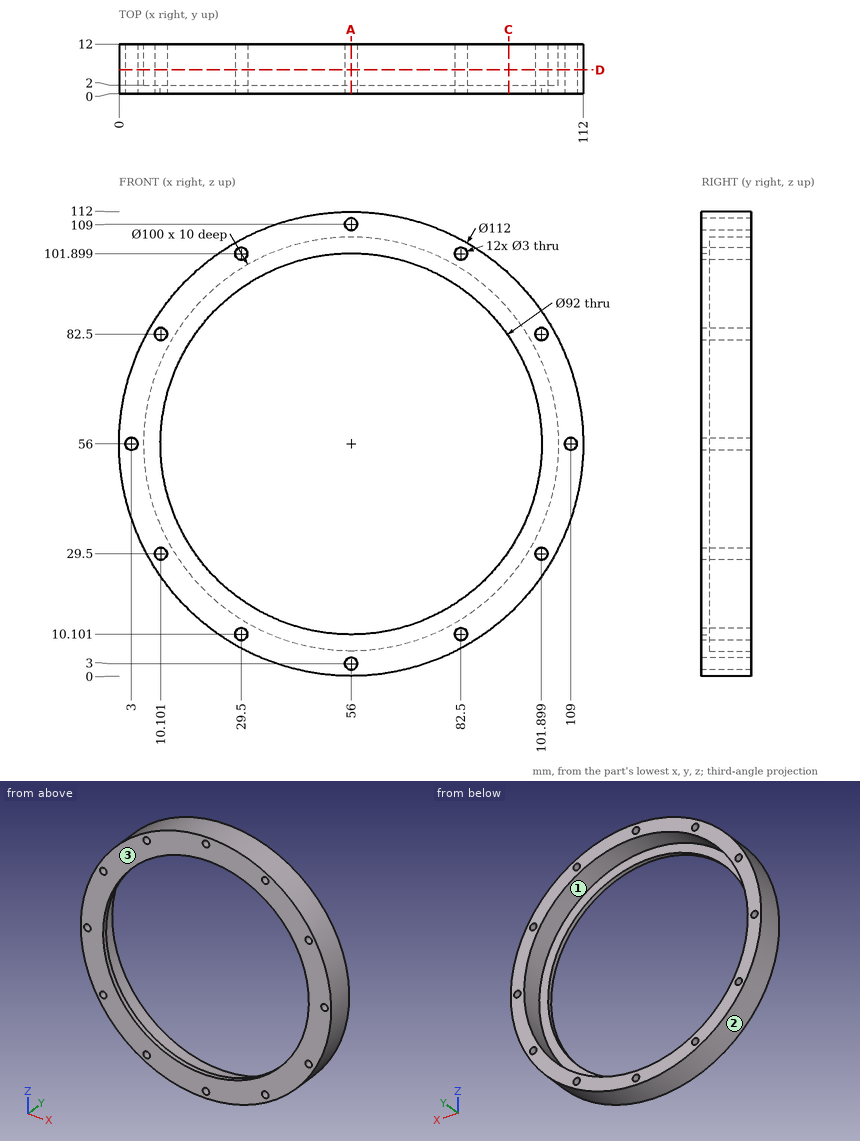
Job drawing, mm, ordinate dimensions from the low corner. One solid piece. Coordinates: 2 decimals unless noted, no trailing zeros. Write each loop counter-clockwise with the first axis right and the second up, starting at its lowest first coordinate (ties: lowest second). Pieces come first, ordered by that corner, then holes.
Item 1: Mould opens along X. For the marked faces 1, 2 and 3 say: released by +X, released by -X, zero draft, split by the parting line, or undercut.
Item 2: Probe line 1 (X direction, y = 7.5, z = 56); line 2 (X direction, y = 11.5, z = 81.5); line 3 (Z direction, x = 82.5, y = 6). List the from-to ranges inside material, lowest first.
Item 3: Pin check, flat tips, straight feed: pin 1 (5 mm diameter, centred on x = 13, y = 8.5, fed in from -Z) (1 decimal); pin 2 (6 mm diameter, centred on y = 10, z = 82.5, fed in from -X); pin 3 (2 mm diameter, centred on x = 32, z = 98, fed in from +Y). Stop position of each tip, or through.
Item 4: Slice it at D-D (y = 5.75). Count the separate pieces of the cut face and the enclosed holes in it, and give its area (3 significant figures).
Item 5: Slice it at C-C (x = 94). Write the cut outline in (y, z), and give its area (3 significant figures).
Item 6: Slice it at A-A (x = 56). Write the cut outline in (y, z).
Results found:
1. face 1: undercut
1. face 2: split by the parting line
1. face 3: zero draft
2. line 1: x = 0 to 1.5, 4.5 to 6, 106 to 107.5, 110.5 to 112
2. line 2: x = 6.14 to 8.98, 11.22 to 12.99, 99.01 to 100.78, 103.02 to 105.86
2. line 3: z = 6.67 to 8.6, 11.6 to 13.6, 98.4 to 100.4, 103.4 to 105.33
3. pin 1: stops at z = 17.3
3. pin 2: stops at x = 5.17
3. pin 3: stops at y = 2
4. separate pieces: 1
4. enclosed holes: 13
4. area: 1,910 mm2
5. outline: (0, 14.87) - (12, 14.87) - (12, 23.5) - (2, 23.5) - (2, 30.08) - (0, 30.08) - close; (0, 81.92) - (2, 81.92) - (2, 88.5) - (12, 88.5) - (12, 97.13) - (0, 97.13) - close
5. area: 234 mm2
6. outline: (0, 0) - (12, 0) - (12, 1.5) - (0, 1.5) - close; (0, 4.5) - (12, 4.5) - (12, 6) - (2, 6) - (2, 10) - (0, 10) - close; (0, 102) - (2, 102) - (2, 106) - (12, 106) - (12, 107.5) - (0, 107.5) - close; (0, 110.5) - (12, 110.5) - (12, 112) - (0, 112) - close
